Solid Edge part; units mm, degrees
sketch "Sketch1" plane through (0, 0, 0) normal (0, 0, 1) x (1, 0, 0)
  circle A0 centre (14.4678, -22.0032) radius 31.75
  circle A1 centre (14.4678, -22.0032) radius 12.7
extrude "Protrusion1" add sketch "Sketch1" against normal blind 6.35
sketch "Sketch2" plane through (0, 0, 0) normal (0, 0, 1) x (1, 0, 0)
  line L0 (58.9178, -53.7532) -> (-17.2822, -53.7532)
  line L1 (-17.2822, -53.7532) -> (-17.2822, 9.7468)
  line L2 (-17.2822, 9.7468) -> (58.9178, 9.7468)
  line L3 (58.9178, 9.7468) -> (58.9178, -53.7532)
extrude "ExtrudedProtrusion_2" add sketch "Sketch2" along normal blind 12.7
sketch "Sketch3" plane through (-17.2822, -22.0032, 6.35) normal (-1, 0, 0) x (0, -1, 0)
  line L0 (25.4, 12.7) -> (-25.4, 12.7)
  line L1 (-25.4, 12.7) -> (-19.05, 6.35)
  line L2 (19.05, 6.35) -> (-19.05, 6.35)
  line L3 (25.4, 12.7) -> (19.05, 6.35)
extrude "ExtrudedProtrusion_3" add sketch "Sketch3" against normal blind 76.2
hole "Hole_1" at (14.4678, -22.0032, 19.05) direction (0, 0, -1) diameter 6.35 end up to next
fillet "Round_1" radius 6.35 4 edges at (-17.2822, -53.7532, 6.35) (-17.2822, 9.7468, 6.35) (58.9178, -53.7532, 6.35) (58.9178, 9.7468, 6.35)
hole "Hole_2" at (-17.2822, 3.3968, 6.35) direction (1, 0, 0) diameter 3.175 depth 50.8 counterbore diameter 6.35 counterbore depth 6.35
hole "Hole1" at (-17.2822, -47.4032, 6.35) direction (1, 0, 0) diameter 3.175 depth 50.8 counterbore diameter 6.35 counterbore depth 6.35
Part model, mm, in its own coordinate system. A direction names the side the tool comes from. Coordinates: 2 decimals unless noted, no trailing zeros. Write each loop counter-clockwise with the first axis right and the second up, starting at its lowest first coordinate (ties: lowest second). Pieces come first, ordered by that corner, then holes.
Item 1: Which spindle directions (+Z, -Z, +X, -X, +Y, -Y) get a long thin tool onto all of the face, cutting with end or side? Do faces 5 (the face through (-14.06, 0.25, 5.94)), 6 (the face through (-10, -46, 0)), 7 (the face through (21, -47, 12.7)), 8 (the face through (21, 3, 12.7)), 9 (the face through (44.752, -12.466, -3.131)). Say none if no direction does.
Item 2: Mould opens along X. For faces 1 (the face through (20.284, -44.273, 15.919)), 2 (the face through (4.39, -29.73, -3.13)), 3 (the face through (57.01, -51.94, 6.44)), 4 (the face through (12, -25, 0)) say: released by +X, released by -X, zero draft, split by the parting line, or undercut.
Item 3: Slice it at C-C (y = -37). Write the cut outline in (x, z).
Item 4: Slice it at B-B (x = -0.5). Count the separate pieces of the cut face and the enclosed holes in it, and give its area (3 significant figures).
Item 5: Probe line 1 (Y direction, x = 24, z = 6.35); line 2 (Y direction, x = -13, z = 6.35); line 3 (Y direction, x = 16.5, z = 6.35). List the from-to ranges inside material, lowest first.
Item 6: Pin check, flat tips, straight feed: pin 1 (5 mm diameter, centred on x = 13, y = -14, fed in from -Z); pin 2 (1.5 mm diameter, centred on x = 4, z = -1.5, fed in from +Y); pin 3 (1.6 mm diameter, centred on y = -47.5, z = 6, fed in from -X). Stop position of each tip, or through.
Item 7: Slice it at A-A (z = -3.5). Write the cut outline in (x, y).
Results found:
1. face 5: -X
1. face 6: -Z, -X, -Y
1. face 7: +X, -X, -Y
1. face 8: +X, -X, +Y
1. face 9: -Z
2. face 1: zero draft
2. face 2: undercut
2. face 3: released by +X
2. face 4: undercut
3. outline: (-17.28, 0) - (-13.52, 0) - (-13.52, -6.35) - (42.45, -6.35) - (42.45, 0) - (58.92, 0) - (58.92, 19.05) - (-17.28, 19.05) - close
4. separate pieces: 1
4. enclosed holes: 2
4. area: 1,430 mm2
5. line 1: y = -53.75 to -48.99, -45.82 to 1.81, 4.98 to 9.75
5. line 2: y = -53.41 to -50.58, -44.23 to 0.22, 6.57 to 9.4
5. line 3: y = -53.75 to -48.99, -45.82 to -24.44, -19.56 to 1.81, 4.98 to 9.75
6. pin 1: stops at z = 0
6. pin 2: stops at y = 8.22
6. pin 3: stops at x = 33.52
7. outline: circle Ø63.5 at (14.47, -22); hole circle Ø25.4 at (14.47, -22)
